Geometry: final body of the model. Coordinates: model frame, mm. Face numbers are marked on the shaded views. A direction names the side the tool comes from. Coordinates: 2 decimals unless noted, no trailing zeros. Write each loop counter-clockwise with the first axis right and the second up, starting at its lowest first coordinate (ties: lowest second). Pieces come first, ordered by that corner, then holes. Notation, with made-up numbers: (77, -37.75) -> (130, -37.75) arc R21 cw to (130, -27.75) -> close; hole circle Ø10 at (-9.5, -37). An arc over 180 degrees is marked (long way). Answer as a JSON object with one key per item and string values. Group by question number.
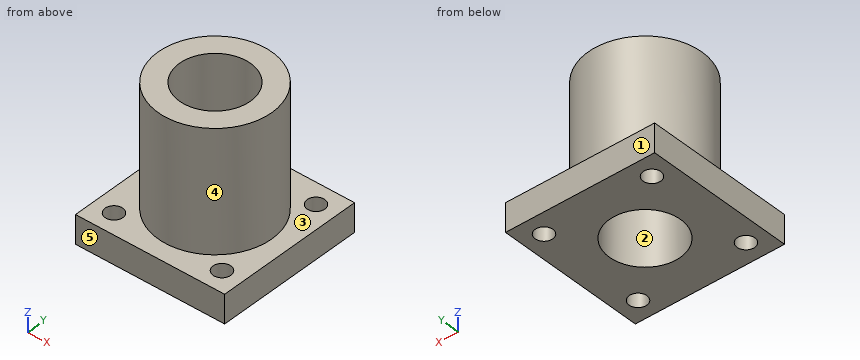
```python
from build123d import *

# Parameters (mm, degrees)
SKETCH_1_W      = 42
SKETCH_1_H      = 42
SKETCH_1_R      = 2.5
SKETCH_1_R_2    = 16
SKETCH_1_R_3    = 10
EXTRUDE_1_DEPTH = 8
SKETCH_1_3_R    = 16
SKETCH_1_3_R_2  = 10
EXTRUDE_2_DEPTH = 42


with BuildPart() as part:
    # Sketch 1 → Extrude 1 (new body)
    # profile 1 of 2: a face of its own
    with BuildSketch(Plane.XY):
        Rectangle(SKETCH_1_W, SKETCH_1_H)
        with Locations((-15.202795796, -15.202795796)):
            Circle(SKETCH_1_R, mode=Mode.SUBTRACT)
        with Locations((15.202795796, -15.202795796)):
            Circle(SKETCH_1_R, mode=Mode.SUBTRACT)
        with Locations((15.202795796, 15.202795796)):
            Circle(SKETCH_1_R, mode=Mode.SUBTRACT)
        with Locations((-15.202795796, 15.202795796)):
            Circle(SKETCH_1_R, mode=Mode.SUBTRACT)
        Circle(SKETCH_1_R_2, mode=Mode.SUBTRACT)
    # profile 2 of 2: a face of its own
    with BuildSketch(Plane.XY):
        Circle(SKETCH_1_R_2)
        Circle(SKETCH_1_R_3, mode=Mode.SUBTRACT)
    extrude(amount=EXTRUDE_1_DEPTH)

    # Sketch 1_3 → Extrude 2 (add)
    with BuildSketch(Plane.XY):
        with Locations(Location((0, 0, 0), (0, 0, 180))):
            Circle(SKETCH_1_3_R)
        Circle(SKETCH_1_3_R_2, mode=Mode.SUBTRACT)
    extrude(amount=EXTRUDE_2_DEPTH)


solid = part.part
```
Item 1: Mould query, pull axis Y, two halves, no side actions, for the marked faces 1, 2 and 3. Classes: +Y half, -Y half, draft (parallel to the pull), parting line (faces both ways), or undercut.
Item 2: Contact query for flat-ended pins moving along their axis: pin 1 (1 mm diameter, centred on x = 3, z = 10.5, fed in from +Y); pin 2 (6 mm diameter, centred on x = 15.2, y = 15.2, fed in from +Z); pin 3 (1 mm diameter, centred on y = 9, z = 17.5, fed in from +X). Output: stop coordinate, or through.
Item 3: Section C-C on x = -13.5. Output: boundary loops of the cut face in (y, z), then the cut area to 3 significant figures.
Item 4: Section D-D on y = -17. Output: boundary loops of the cut face in (x, z), then the cut area to 3 significant figures.
Item 5: Set-up query: the marked faces 4 and 5. Return all of +Z, -Z, +X, -X, +Y, -Y with unobstructed straight access to the full face (end or side cutting, diameter ignored); none if empty.
Item 6: Section A-A on y = 0. Output: boundary loops of the cut face in (x, z).
Item 7: Ray query, L1, parallel to X at y = -13.5, z = 7; L2, parallel to X at y = 14, z = 4.5; L3, parallel to X at y = 0.5, z = 35.5. Return the intervals inside material, ascending. Write a range as [from, to].
Answer sheet:
{
 "1": {"face 1": "+Y half", "face 2": "undercut", "face 3": "draft"},
 "2": {"pin 1": "stops at y = 15.8", "pin 2": "stops at z = 8", "pin 3": "stops at x = 13.56"},
 "3": {"outline": "(-21, 0) -> (-17.03, 0) -> (-17.03, 8) -> (-21, 8) -> close; (-13.37, 0) -> (13.37, 0) -> (13.37, 8) -> (8.59, 8) -> (8.59, 42) -> (-8.59, 42) -> (-8.59, 8) -> (-13.37, 8) -> close; (17.03, 0) -> (21, 0) -> (21, 8) -> (17.03, 8) -> close", "area": "861 mm^2"},
 "4": {"outline": "(-21, 0) -> (-16.94, 0) -> (-16.94, 8) -> (-21, 8) -> close; (-13.46, 0) -> (13.46, 0) -> (13.46, 8) -> (-13.46, 8) -> close; (16.94, 0) -> (21, 0) -> (21, 8) -> (16.94, 8) -> close", "area": "280 mm^2"},
 "5": {"face 4": "+Z", "face 5": "+Z, -Z, +X, -X, -Y"},
 "6": {"outline": "(-21, 0) -> (-10, 0) -> (-10, 42) -> (-16, 42) -> (-16, 8) -> (-21, 8) -> close; (10, 0) -> (21, 0) -> (21, 8) -> (16, 8) -> (16, 42) -> (10, 42) -> close"},
 "7": {"L1": "x = [-21, -17.03], [-13.37, 13.37], [17.03, 21]", "L2": "x = [-21, -17.39], [-13.01, 13.01], [17.39, 21]", "L3": "x = [-15.99, -9.99], [9.99, 15.99]"}
}
